Solid Edge part; units mm, degrees
sketch "Sketch1" plane through (0, 0, 0) normal (0, -1, 0) x (1, 0, 0)
  line L0 (-20, 5) -> (-20, 0)
  line L1 (-20, 0) -> (20, 0)
  line L2 (20, 0) -> (20, 5)
  line L3 (20, 5) -> (14, 5)
  line L4 (14, 5) -> (10, 20)
  line L5 (10, 20) -> (-10, 20)
  line L6 (-10, 20) -> (-14, 5)
  line L7 (-14, 5) -> (-20, 5)
  dimension "D1" = 10
  dimension "D2" = 20
  dimension "D3" = 20
  dimension "D4" = 14
extrude "Protrusion1" add sketch "Sketch1" along normal mid plane 10
fillet "rounds" radius 3 2 edges at (10, 0, 20) (-10, 0, 20)
hole "Hole1" at (0, 5, 13.75) direction (0, -1, 0) diameter 3.4 end up to next counterbore diameter 6.5 counterbore depth 3.5
hole "Hole2" at (8.75, 5, 5) direction (0, -1, 0) diameter 3.4 end up to next counterbore diameter 6.5 counterbore depth 3.5
hole "Hole3" at (-8.75, 5, 5) direction (0, -1, 0) diameter 3.4 end up to next counterbore diameter 6.5 counterbore depth 3.5
hole "Hole4" at (-17, 0, 5) direction (0, 0, -1) diameter 3.2 end up to next start chamfer 0.3 start chamfer angle 45 end chamfer 0.3 end chamfer angle 45
hole "Hole5" at (17, 0, 5) direction (0, 0, -1) diameter 3.2 end up to next start chamfer 0.3 start chamfer angle 45 end chamfer 0.3 end chamfer angle 45
properties material "Polyethylene, low density"
For this review, take the finished solid that the model builds, in its own axes (mm). A direction names the side the tool comes from. Coordinates: 2 decimals unless noted, no trailing zeros. Order: outer loops, then holes, each group sorted by start corner. A loop starts at its lowest first (then second) coordinate and runs counter-clockwise, first axis right, second up. Notation, with made-up numbers: (6, 26.25) -> (30, 26.25) arc R34 ccw to (30, 65.25) -> close; hole circle Ø1 at (-21.75, 75.25). An arc over 180 degrees is marked (long way). Return JSON: item names as keys, results as strings.
1. The part is to be moulded in two halves that separate along Z. For faces 4 (the flat face through (17, 2.3, 5)), 5 (the flat face through (0, -5, 8)), 6 (the flat face through (-7, 1.5, 6)), say which applies: +Z half, -Z half, draft (parallel to the pull), parting line (faces both ways), or undercut.
Answer block:
{"face 4": "+Z half", "face 5": "draft", "face 6": "undercut"}
2. We need section B-B on y = 4.25. Write out the cut boundary in (x, z), and give its area (3 significant figures).
Answer block:
{"outline": "(-20, 0) -> (20, 0) -> (20, 5) -> (14, 5) -> (10.59, 17.77) arc R3 ccw to (7.7, 20) -> (-7.7, 20) arc R3 ccw to (-10.59, 17.77) -> (-14, 5) -> (-20, 5) -> close; hole circle Ø6.5 at (-8.75, 5); hole circle Ø6.5 at (0, 13.75); hole circle Ø6.5 at (8.75, 5)", "area": "458 mm²"}
3. Machinability: for faces 1 (the cylindrical face through (-11.49, 3.23, 6.75)), 2 (the flat face through (-17, 2.3, 5)), 3 (the cylindrical face through (-10.26, -1.7, 5.78)), which of the approach directions +Z, -Z, +X, -X, +Y, -Y give a long, thin tool a straight path to every point of the face, cutting with its end or side? Answer none if there is none.
Answer block:
{"face 1": "+Y", "face 2": "+Z, -X, +Y, -Y", "face 3": "+Y, -Y"}
4. We need section D-D on z = 14.25. Write out the cut boundary in (x, y), and give its area (3 significant figures).
Answer block:
{"outline": "(-11.53, -5) -> (-1.62, -5) -> (-1.62, 1.5) -> (-3.21, 1.5) -> (-3.21, 5) -> (-11.53, 5) -> close; (1.62, -5) -> (11.53, -5) -> (11.53, 5) -> (3.21, 5) -> (3.21, 1.5) -> (1.62, 1.5) -> close", "area": "187 mm²"}
5. For line 1 (X direction, y = 0, z = 1.45); line 2 (Z direction, x = 0, y = 2.6); line 3 (X direction, y = -2.5, z = 3.5), list the stretches that pass through material, from the lowest coordinate up. Write a range as from..to.
Answer block:
{"line 1": "-20..-18.6, -15.4..15.4, 18.6..20", "line 2": "0..10.5, 17..20", "line 3": "-20..-9.55, -7.95..7.95, 9.55..20"}
6. For pin 1 Ø2 at (y, z) = (0, 16.5) entering from +X; pin 2 Ø5 at (x, z) = (0, 13.75) entering from +Y; pin 3 Ø4 at (y, z) = (-2, 11.5) entering from +X; pin 4 Ø2.5 at (x, z) = (8.75, 5) entering from -Y, all flat-tipped, find the tip position at first contact; note any pin that passes through.
Answer block:
{"pin 1": "x = 11.2", "pin 2": "y = 1.5", "pin 3": "x = 12.8", "pin 4": "through"}
7. We need section A-A on y = 0. State how many separate pieces and enclosed holes the cut face has, and give its area (3 significant figures).
Answer block:
{"separate pieces": "3", "enclosed holes": "3", "area": "498 mm²"}
8. We need section C-C on x = -17. Write out the cut boundary in (y, z), and give its area (3 significant figures).
Answer block:
{"outline": "(-5, 0) -> (-1.9, 0) -> (-1.6, 0.3) -> (-1.6, 4.7) -> (-1.9, 5) -> (-5, 5) -> close; (1.6, 0.3) -> (1.9, 0) -> (5, 0) -> (5, 5) -> (1.9, 5) -> (1.6, 4.7) -> close", "area": "33.8 mm²"}
